Here's how the part is built. I have some questions about the finished solid (model axes, mm). Round coordinates to 2 decimals unless told otherwise and drop trailing zeros. Loops run counter-clockwise (first coordinate to the right, second up) from the corner with the lowest first, then second, coordinate; pieces in that order, holes last. Notation, with made-up numbers: M 22.25,6 L 42.25,6 A22 cw 42.25,12 Z; hole C 27,30 d3. An arc over 180 degrees is marked long. Answer as a JSON object with one key per item and string values.
from build123d import *

# Parameters (mm, degrees)
F0_W     = 76.2
F0_H     = 50.8
F1_DEPTH = 25.4
F2_R     = 6.35
F3_DEPTH = 25.401
F4_R     = 6.35
F5_DEPTH = 76.201
F6_R     = 6.35
F7_DEPTH = 50.801
F8_R     = 3.175


with BuildPart() as f1:
    # F0 (on Front) → F1 (new body)
    with BuildSketch(Plane.XZ):
        with Locations((38.1, 25.4)):
            Rectangle(F0_W, F0_H)
    extrude(amount=F1_DEPTH)

    # F2 (on face) → F3 (cut, through all)
    with BuildSketch(Plane.XZ.offset(25.4)):
        with Locations((38.1, 25.4)):
            Circle(F2_R)
    extrude(amount=-F3_DEPTH, mode=Mode.SUBTRACT)

    # F4 (on face) → F5 (cut, through all)
    with BuildSketch(Plane(origin=(0, 0, 0), x_dir=(0, -1, 0), z_dir=(-1, 0, 0))):
        with Locations((12.7, 25.4)):
            Circle(F4_R)
    extrude(amount=-F5_DEPTH, mode=Mode.SUBTRACT)

    # F6 (on face) → F7 (cut, through all)
    with BuildSketch(Plane(origin=(0, 0, 0), x_dir=(1, 0, 0), z_dir=(0, 0, -1))):
        with Locations((38.1, 12.7)):
            Circle(F6_R)
    extrude(amount=-F7_DEPTH, mode=Mode.SUBTRACT)

    # F8
    f8_edges = [f1.edges().sort_by_distance(p)[0] for p in [
        (0, -12.7, 50.8),
        (0, -25.4, 25.4),
        (38.1, -25.4, 0),
        (76.2, -25.4, 25.4),
        (76.2, -12.7, 50.8),
        (76.2, 0, 25.4),
        (38.1, -25.4, 50.8),
        (38.1, 0, 50.8),
        (38.1, 0, 0),
        (0, -12.7, 0),
        (0, 0, 25.4),
        (76.2, -12.7, 0),
    ]]
    fillet(f8_edges, radius=F8_R)


solid = f1.part
Item 1: I want a section at A-A on z = 25.4. List the corners of the cut face in (x, y) for me (3 decimals), plus the area to 3 significant figures.
Solution:
{"outline": "M 0,-22.225 A3.175 ccw 3.175,-25.4 L 31.75,-25.4 L 31.75,-19.05 L 0,-19.05 Z; M 0,-6.35 L 31.75,-6.35 L 31.75,0 L 3.175,0 A3.175 ccw 0,-3.175 Z; M 44.45,-25.4 L 73.025,-25.4 A3.175 ccw 76.2,-22.225 L 76.2,-19.05 L 44.45,-19.05 Z; M 44.45,-6.35 L 76.2,-6.35 L 76.2,-3.175 A3.175 ccw 73.025,0 L 44.45,0 Z", "area": "798 mm2"}
Item 2: I want a section at B-B on y = -12.7. List the corners of the cut face in (x, z) for me (3 decimals), plus the area to 3 significant figures.
Solution:
{"outline": "M 0,3.175 A3.175 ccw 3.175,0 L 31.75,0 L 31.75,19.05 L 0,19.05 Z; M 0,31.75 L 31.75,31.75 L 31.75,50.8 L 3.175,50.8 A3.175 ccw 0,47.625 Z; M 44.45,0 L 73.025,0 A3.175 ccw 76.2,3.175 L 76.2,19.05 L 44.45,19.05 Z; M 44.45,31.75 L 76.2,31.75 L 76.2,47.625 A3.175 ccw 73.025,50.8 L 44.45,50.8 Z", "area": "2,410 mm2"}
Item 3: I want a section at D-D on x = 69.5. List the corners of the cut face in (y, z) for me (3 decimals), plus the area to 3 significant figures.
Solution:
{"outline": "M -25.4,3.175 A3.175 ccw -22.225,0 L -3.175,0 A3.175 ccw 0,3.175 L 0,47.625 A3.175 ccw -3.175,50.8 L -22.225,50.8 A3.175 ccw -25.4,47.625 Z; hole C -12.7,25.4 d12.7", "area": "1,150 mm2"}
Item 4: If I drill on L1, parallel to Z at x = 9, y = -12.7; L2, parallel to Y at x = 38, z = 10; L3, parallel to X at y = -12.7, z = 45, over which ranges is the centre line in solid material (lowest first)? Write a range as from..to.
Solution:
{"L1": "z = 0..19.05, 31.75..50.8", "L2": "y = -25.4..-19.05, -6.35..0", "L3": "x = 0..31.75, 44.45..76.2"}
Item 5: We'd pull the mould along Y, two halves only. Please class faces 1 (the face through (38, -6, 0)), 2 (the face through (59.16, -18.566, 22.968)), 3 (the face through (31.756, -12.979, 10.309)), 4 (the face through (38.59, -24.45, 0.91)): +Y half, -Y half, draft (parallel to the pull), parting line (faces both ways), or undercut.
Solution:
{"face 1": "draft", "face 2": "undercut", "face 3": "undercut", "face 4": "-Y half"}
Item 6: I want a section at C-C on z = 41. List the corners of the cut face in (x, y) for me (3 decimals), plus the area to 3 significant figures.
Solution:
{"outline": "M 0,-22.225 A3.175 ccw 3.175,-25.4 L 73.025,-25.4 A3.175 ccw 76.2,-22.225 L 76.2,-3.175 A3.175 ccw 73.025,0 L 3.175,0 A3.175 ccw 0,-3.175 Z; hole C 38.1,-12.7 d12.7", "area": "1,800 mm2"}
Item 7: For P1, Ø10, axis at x = 38.1, z = 25.4, coming from the -Y side, with a flat end and sliding along its axis, tell me the tip position at first contact or that it passes through.
Solution:
{"P1": "passes through"}
